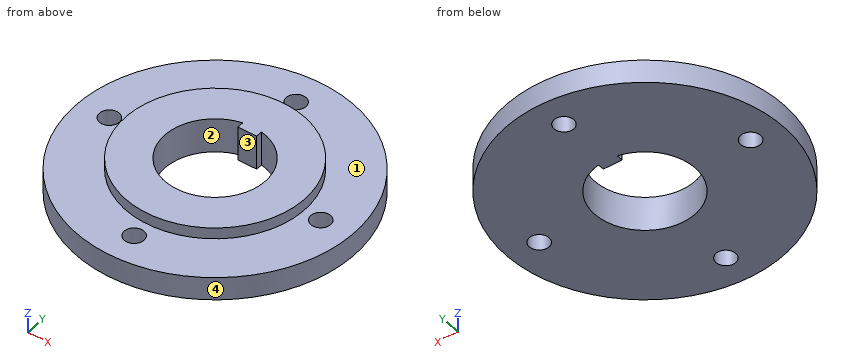
from build123d import *

# Parameters (mm, degrees)
SKETCH_R     = 42
PAD_DEPTH    = 7
SKETCH003_R  = 27
PAD001_DEPTH = 3.4
SKETCH004_R  = 3
HOLE_DEPTH   = 25


with BuildPart() as part:
    # Sketch → Pad (new body)
    with BuildSketch(Plane.XY):
        Circle(SKETCH_R)
        with BuildLine():
            Line((-2.9, 14.895322), (-2.9, 12.895322))
            Line((-2.9, 12.895322), (2.9, 12.895322))
            Line((2.9, 12.895322), (2.9, 14.895322))
            ThreePointArc((-2.9, 14.895322), (0, -15.175), (2.9, 14.895322))
        make_face(mode=Mode.SUBTRACT)
    extrude(amount=PAD_DEPTH)

    # Sketch003 (on Face7 of Pad) → Pad001 (join)
    with BuildSketch(Plane.XY.offset(7)):
        Circle(SKETCH003_R)
        with BuildLine():
            ThreePointArc((-2.9, 14.895322), (0, -15.175), (2.9, 14.895322))
            Line((2.9, 12.895322), (2.9, 14.895322))
            Line((-2.9, 12.895322), (2.9, 12.895322))
            Line((-2.9, 14.895322), (-2.9, 12.895322))
        make_face(mode=Mode.SUBTRACT)
    extrude(amount=PAD001_DEPTH)

    # Sketch004 (on Face3 of Pad001) → Hole (cut)
    with BuildSketch(Plane.XY.offset(7)):
        with Locations((0, 32.5)):
            Circle(SKETCH004_R)
        with Locations((0, -32.5)):
            Circle(SKETCH004_R)
        with Locations((32.5, 0)):
            Circle(SKETCH004_R)
        with Locations((-32.5, 0)):
            Circle(SKETCH004_R)
    extrude(amount=-HOLE_DEPTH, mode=Mode.SUBTRACT)


solid = part.part
Check sheet for the modelled part. Datum: model origin and axes. Units: mm. Face numbers are marked on the shaded views. Round coordinates to 2 decimals unless told otherwise and drop trailing zeros. Order: outer loops, then holes, each group sorted by start corner. A loop starts at its lowest first (then second) coordinate and runs counter-clockwise, first axis right, second up.
Q1. Cross-section at C-C, the plane x = -30.5. Enter the section's corners in (y, z), plus the area to 3 significant figures.
Filled sheet:
outline: (-28.87, 0) - (-2.24, 0) - (-2.24, 7) - (-28.87, 7) - close; (2.24, 0) - (28.87, 0) - (28.87, 7) - (2.24, 7) - close
area: 373 mm2
Q2. Cross-section at B-B, the plane y = 32.5. Enter the section's corners in (x, z), plus the area to 3 significant figures.
Filled sheet:
outline: (-26.6, 0) - (-3, 0) - (-3, 7) - (-26.6, 7) - close; (3, 0) - (26.6, 0) - (26.6, 7) - (3, 7) - close
area: 330 mm2
Q3. Cross-section at A-A, the plane z = 6. Enter the section's corners in (x, y) (3 decimals), plus the area to 3 significant figures.
Filled sheet:
outline: circle Ø84 at (0, 0); hole circle Ø6 at (-32.5, 0); hole circle Ø6 at (0, -32.5); hole circle Ø6 at (0, 32.5); hole (-2.9, 12.895) - (-2.9, 14.895) arc R15.175 ccw (long way) to (2.9, 14.895) - (2.9, 12.895) - close; hole circle Ø6 at (32.5, 0)
area: 4,720 mm2
Q4. Cross-section at D-D, the plane x = 26. Enter the section's corners in (y, z).
Filled sheet:
outline: (-32.98, 0) - (32.98, 0) - (32.98, 7) - (7.28, 7) - (7.28, 10.4) - (-7.28, 10.4) - (-7.28, 7) - (-32.98, 7) - close
Q5. Scan lines: L1, parallel to Y at x = 0, z = 2.25 (3 decimals); L2, parallel to X at y = -2, z = 3.75; L3, parallel to X at y = -0.5, z = 8. Record each from-to range of solid material in increasing order.
Filled sheet:
L1: y = -42 to -35.5, -29.5 to -15.175, 12.895 to 29.5, 35.5 to 42
L2: x = -41.95 to -34.74, -30.26 to -15.04, 15.04 to 30.26, 34.74 to 41.95
L3: x = -27 to -15.17, 15.17 to 27
Q6. Draft check along Y on the marked faces 1, 2, 3 and 4. Enter one of: pulls with the +Y half, pulls with the -Y half, needs draft (parallel to the pull), parting line crosses it, or undercut.
Filled sheet:
face 1: needs draft
face 2: undercut
face 3: undercut
face 4: parting line crosses it
Q7. Depth check by flat-ended pin: P1, Ø4, axis at x = 32, y = 9.5, coming from the +Z side; P2, Ø1.7, axis at x = -1.5, z = 3, coming from the -Y side (3 decimals); P3, Ø2, axis at y = 29, z = 7.5, coming from the -X side. Enter the tip coordinate at first touch or a pass-through.
Filled sheet:
P1: stops at z = 7
P2: stops at y = -41.995
P3: stops at x = -31.18
